Geometry check sheet. Reference: the model listing, model coordinates, mm. Face numbers are marked on the shaded views. A direction names the side the tool comes from. Give positions to 0.01 mm unless a question says otherwise; leave off trailing zeros. Write each loop counter-clockwise with the first axis right and the second up, starting at its lowest first coordinate (ties: lowest second). Pieces come first, ordered by that corner, then holes. Notation, with made-up numbers: M -39,-32.75 L 5,-32.75 A14 cw 5,-10.75 Z; hole C 1.5,-33 d9. An arc over 180 degrees is marked long. Write each question's results on one line, items separated by ' | '.
Autodesk Inventor part; units mm, degrees
ref_plane "YZ Plane" through (0, 0, 0) normal (1, 0, 0) x (0, 1, 0)
ref_plane "XZ Plane" through (0, 0, 0) normal (0, 1, 0) x (-1, 0, 0)
ref_plane "XY Plane" through (0, 0, 0) normal (0, 0, 1) x (1, 0, 0)
sketch "Sketch1" plane through (0, 0, 0) normal (0, 0, 1) x (1, 0, 0)
  line L0 (0, 40) -> (0, 0)
  line L1 (0, 0) -> (6, 0)
  line L2 (6, 0) -> (6, 8.2)
  line L3 (6, 8.2) -> (22, 8.2)
  line L4 (22, 8.2) -> (22, 0)
  line L5 (22, 0) -> (28, 0)
  line L6 (28, 0) -> (28, 40)
  line L7 (28, 40) -> (0, 40)
  dimension "d0" = 6
  dimension "d1" = 6
  dimension "d2" = 16
  dimension "d3" = 40
  dimension "d4" = 8.2
extrude "Extrusion1" add sketch "Sketch1" against normal blind 8.2
sketch "Sketch2" plane through (28, 0, 0) normal (1, 0, 0) x (0, 0, -1)
  circle A0 centre (4.1, 4.1) radius 2.05
  line L0 (0, 0) -> (8.2, 0)
  line L1 (0, 0) -> (8.2, 0)
  point P0 (4.1, 0)
  dimension "d7" = 4.1
  dimension "d8" = 4.1
  dimension "d9" = 8.2
extrude "Extrusion2" cut sketch "Sketch2" against normal through all
fillet "Fillet1" radius 4.1 5 edges at (25, 0, 0) (3, 0, 0) (3, 0, -8.2) (25, 0, -8.2) (14, 8.2, -8.2)
sketch "Sketch3" plane through (0, 0, -8.2) normal (0, 0, -1) x (-1, 0, 0)
  line L0 (0, 40) -> (-28, 40)
  line L1 (-20, 40) -> (-16, 40)
  line L2 (-16, 40) -> (-16, 32)
  line L3 (-16, 32) -> (-20, 32)
  line L4 (-20, 32) -> (-20, 40)
  line L5 (-12, 40) -> (-8, 40)
  line L6 (-8, 40) -> (-8, 32)
  line L7 (-8, 32) -> (-12, 32)
  line L8 (-12, 32) -> (-12, 40)
  point P0 (0, 0)
  point P1 (-14, 40)
  dimension "d13" = 4
  dimension "d14" = 4
  dimension "d15" = 4
  dimension "d16" = 2
  dimension "d17" = 8
extrude "Extrusion3" add sketch "Sketch3" along normal blind 8.2
sketch "Sketch4" plane through (20, 32, -8.2) normal (1, 0, 0) x (0, 0, -1)
  circle A0 centre (4.2, 4) radius 2.05
  line L0 (8.2, 8) -> (8.2, 0)
  point P0 (-8.2, -32)
  dimension "d20" = 4.1
  dimension "d21" = 8
  dimension "d22" = 4
  dimension "d23" = 4
extrude "Extrusion4" cut sketch "Sketch4" against normal through all
fillet "Fillet2" radius 4.1 6 edges at (10, 40, -16.4) (18, 40, -16.4) (18, 32, -16.4) (10, 32, -16.4) (18, 32, -8.2) (10, 32, -8.2)
fillet "Fillet3" radius 4.1 4 edges at (14, 40, 0) (4, 40, -8.2) (14, 40, -8.2) (24, 40, -8.2)
sketch "Sketch5" plane through (0, 0, 0) normal (0, 0, 1) x (1, 0, 0)
  circle A0 centre (4, 34.1) radius 1.3
  line L0 (0, 35.9) -> (28, 35.9) construction
  line L1 (0, 35.9) -> (0, 4.1) construction
  circle A1 centre (4, 14.1) radius 1.3
  circle A2 centre (24, 34.1) radius 1.3
  circle A3 centre (24, 14.1) radius 1.3
  line L2 (28, 4.1) -> (28, 35.9) construction
  line L3 (6, 12.3) -> (22, 12.3) construction
  point P0 (0, 0)
  point P1 (14, 35.9)
  dimension "d30" = 20
  dimension "d33" = 20
  dimension "d36" = 1.8
  dimension "d37" = 10
  dimension "d38" = 2.6
  dimension "d42" = 23.6
extrude "Extrusion5" cut sketch "Sketch5" against normal up to surface (8.2 mm away)
equation "\"d0\" = d1"
equation "\"d4\" = 2 * arm_rod_diam"
equation "\"d5\" = 2 * arm_rod_diam"
equation "\"d7\" = arm_rod_diam"
equation "\"d8\" = 0.5 * d9"
equation "\"d12\" = arm_rod_diam"
equation "\"d13\" = d14"
equation "\"d18\" = 2 * arm_rod_diam"
equation "\"d20\" = arm_rod_diam"
equation "\"d22\" = 0.5 * d21"
equation "\"d23\" = d22"
equation "\"d26\" = arm_rod_diam"
equation "\"d27\" = arm_rod_diam"
equation "\"d36\" = -0.5 * d30 + 0.5 * d42"
equation "\"arm_rod_diam\" = 4.1"
properties part number "camera_arm" material "ABS Plastic"
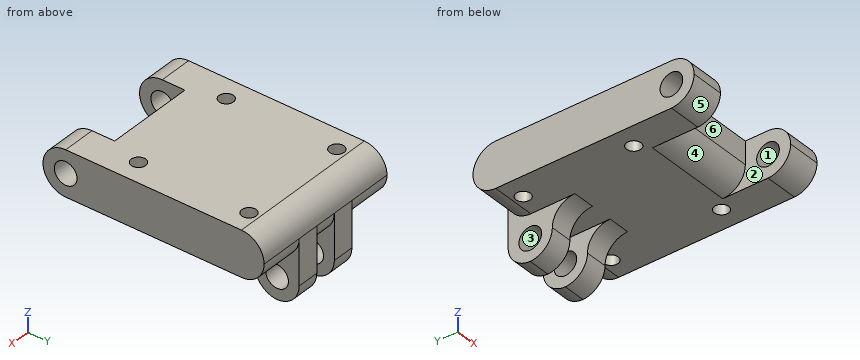
Q1. Section check B-B (y = 14.1). Enter the section's corners in (x, z).
Answer key:
outline: M 0,-8.2 L 2.7,-8.2 L 2.7,0 L 0,0 Z; M 5.3,-8.2 L 22.7,-8.2 L 22.7,0 L 5.3,0 Z; M 25.3,-8.2 L 28,-8.2 L 28,0 L 25.3,0 Z
Q2. Section check A-A (x = 4). State how many separate pieces and enclosed holes the cut face has, then the cut area to 3 significant figures.
Answer key:
separate pieces: 3 | enclosed holes: 1 | area: 258 mm2
Q3. Release check for a two-part mould opening along Y. For the marked faces 1, 2, 3 and 4 record: released by +Y, released by -Y, zero draft, split by the parting line, or undercut.
Answer key:
face 1: undercut | face 2: zero draft | face 3: undercut | face 4: released by -Y
Q4. Access from +Z, -Z, +X, -X, +Y, -Y to the whole of each face (thin tool, end or side, straight path). Record for the marked faces 5 and 6.
Answer key:
face 5: -Z, +X, -X, -Y | face 6: +Z, -Z, -Y
Q5. Depth check by flat-ended pin: P1, Ø5, axis at x = 12.5, y = 20, coming from the +Z side; P2, Ø4, axis at x = 8, z = -14, coming from the -Y side; P3, Ø6, axis at y = 32, z = -12.5, coming from the -X side; P4, Ø1, axis at x = 14.5, y = 30.5, coming from the -Z side. Enter the tip coordinate at first touch or a pass-through.
Answer key:
P1: stops at z = 0 | P2: stops at y = 31.99 | P3: stops at x = 8 | P4: stops at z = -8.2
Q6. Section check D-D (y = 5). Enter the section's corners in (x, z).
Answer key:
outline: M 0,-8.2 L 6,-8.2 L 6,-5.94 L 0,-5.94 Z; M 0,-2.26 L 6,-2.26 L 6,0 L 0,0 Z; M 22,-8.2 L 28,-8.2 L 28,-5.94 L 22,-5.94 Z; M 22,-2.26 L 28,-2.26 L 28,0 L 22,0 Z
Q7. Material ranges on probe 1 along Y at (x, z) = (4, -2.5); probe 2 along Y at (x, z) = (4, -3.5); probe 3 along X at (y, z) = (35, -10), recorded low to high. Write a range as [from, to].
Answer key:
probe 1: y = [0.33, 2.82], [5.38, 12.8], [15.4, 32.8], [35.4, 39.67] | probe 2: y = [0.04, 2.14], [6.06, 12.8], [15.4, 32.8], [35.4, 39.96] | probe 3: x = [8, 12], [16, 20]
